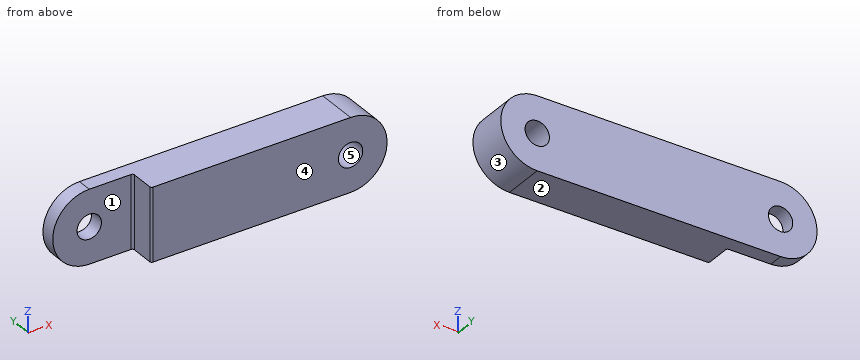
```python
from build123d import *

# Parameters (mm, degrees)
SKETCH1_R           = 2.4
BOSS_EXTRUDE1_DEPTH = 15
SKETCH2_R           = 2.4
CUT_EXTRUDE1_DEPTH  = 12
SKETCH3_W           = 81.763751064
SKETCH3_H           = 26.290001284
CUT_EXTRUDE2_DEPTH  = 5
SCALE1_SCALE        = 0.8
SKETCH4_R           = 2
CUT_EXTRUDE3_DEPTH  = 52.087489074
SKETCH5_W           = 42.014746782
SKETCH5_H           = 19.111045429
CUT_EXTRUDE4_DEPTH  = 1.2
FILLET1_R           = 0.3
FILLET3_R           = 0.3


with BuildPart() as part:
    # Sketch1 → Boss-Extrude1 (new body)
    with BuildSketch(Plane(origin=(0, 0, 0), x_dir=(1, 0, 0), z_dir=(0, 1, 0))):
        with BuildLine():
            Line((-50, 7.5), (0, 7.5))
            ThreePointArc((0, 7.5), (7.5, 0), (0, -7.5))
            Line((0, -7.5), (-50, -7.5))
            ThreePointArc((-50, -7.5), (-57.5, 0), (-50, 7.5))
        make_face()
        with Locations(Location((-50, 0, 0), (0, 0, 270))):
            Circle(SKETCH1_R, mode=Mode.SUBTRACT)
        with Locations(Location((0, 0, 0), (0, 0, 270))):
            Circle(SKETCH1_R, mode=Mode.SUBTRACT)
    extrude(amount=BOSS_EXTRUDE1_DEPTH)

    # Sketch2 → Cut-Extrude1 (cut)
    with BuildSketch(Plane(origin=(0, 0, 0), x_dir=(1, 0, 0), z_dir=(0, 1, 0))):
        with BuildLine():
            Line((-50, 7.5), (-41, 7.5))
            Line((-41, 7.5), (-41, -7.5))
            Line((-41, -7.5), (-50, -7.5))
            ThreePointArc((-50, -7.5), (-57.5, 0), (-50, 7.5))
        make_face()
        with Locations(Location((-50, 0, 0), (0, 0, 270))):
            Circle(SKETCH2_R, mode=Mode.SUBTRACT)
    extrude(amount=CUT_EXTRUDE1_DEPTH, mode=Mode.SUBTRACT)

    # Sketch3 → Cut-Extrude2 (cut)
    with BuildSketch(Plane.XZ):
        with Locations((-24.1072482, 0)):
            Rectangle(SKETCH3_W, SKETCH3_H)
    extrude(amount=-CUT_EXTRUDE2_DEPTH, mode=Mode.SUBTRACT)


with BuildPart() as part_1:
    # Scale1: scaled about (-20.496084793, 10.28858221, 0)
    add(part.part.scale(SCALE1_SCALE).moved(Location((-4.099216959, 2.057716442, 0))))

    # Sketch4 → Cut-Extrude3 (cut, through all)
    with BuildSketch(Plane(origin=(0, 14.057716442, 0), x_dir=(1, 0, 0), z_dir=(0, 1, 0))):
        with Locations(Location((-44.099216959, 0, 0), (0, 0, 270))):
            Circle(SKETCH4_R)
        with Locations(Location((-4.099216959, 0, 0), (0, 0, 270))):
            Circle(SKETCH4_R)
    extrude(amount=-CUT_EXTRUDE3_DEPTH, mode=Mode.SUBTRACT)

    # Sketch5 → Cut-Extrude4 (cut)
    with BuildSketch(Plane.XZ.offset(-6.057716442)):
        with Locations((-17.942307993, -0.717456632)):
            Rectangle(SKETCH5_W, SKETCH5_H)
    extrude(amount=-CUT_EXTRUDE4_DEPTH, mode=Mode.SUBTRACT)

    # Fillet1
    fillet1_edges = [part_1.edges().sort_by_distance(p)[0] for p in [
        (-36.899216959, 11.657716442, 0),
    ]]
    fillet(fillet1_edges, radius=FILLET1_R)

    # Fillet3
    fillet3_edges = [part_1.edges().sort_by_distance(p)[0] for p in [
        (-36.899216959, 7.257716442, 0),
    ]]
    fillet(fillet3_edges, radius=FILLET3_R)


solid = part_1.part
```
Model file for the job. Use its own axes, mm. Face numbers are marked on the shaded views. A direction names the side the tool comes from. Give positions to 0.01 mm unless a question says otherwise; leave off trailing zeros. Order: outer loops, then holes, each group sorted by start corner. A loop starts at its lowest first (then second) coordinate and runs counter-clockwise, first axis right, second up.
1) Saw through at D-D, the plane z = -4.75. Write the cut outline in (x, y), then the cut area to 3 significant figures.
2) 3-axis set-ups, long thin cutter, end or side, ignore diameter. For the marked faces 1 and 2: which of +Z, -Z, +X, -X, +Y, -Y reach the whole face in a straight line?
3) Pin check, flat tips, straight feed: pin 1 (2.5 mm diameter, centred on x = -4.1, z = 0, fed in from +Y); pin 2 (1.5 mm diameter, centred on y = 10.5, z = -1.5, fed in from +X); pin 3 (6.5 mm diameter, centred on x = -44.1, z = 0, fed in from -Y); pin 4 (1.1 mm diameter, centred on y = 9, z = -2.5, fed in from -X). Stop position of each tip, or through.
4) Saw through at B-B, the plane y = 8.5. Write the cut outline in (x, z).
5) Saw through at A-A, the plane z = 0. Write the cut outline in (x, y), then the cut area to 3 significant figures.
6) Mould opens along X. For the marked faces 3, 4 and 5 say: +X half, -X half, draft (parallel to the pull), parting line (faces both ways), or undercut.
7) Wall check: probe 1 along X at (y, z) = (13.3, 0); probe 2 along X at (y, z) = (7.75, 0); probe 3 along Y at (x, z) = (-41, -2). Give the ranges that are in metal, low to high.
8) Saw through at C-C, the plane y = 13.5. Write the cut outline in (x, z), then the cut area to 3 significant figures.
Computed:
1. outline: (-47.76, 11.66) - (-37.2, 11.66) arc R0.3 cw to (-36.9, 11.36) - (-36.9, 7.56) arc R0.3 ccw to (-36.6, 7.26) - (-0.43, 7.26) - (-0.43, 14.06) - (-47.76, 14.06) - close
1. area: 274 mm2
2. face 1: +Z, -Z, -X, -Y
2. face 2: -Z, +X, -X, +Y, -Y
3. pin 1: passes through
3. pin 2: stops at x = 1.85
3. pin 3: stops at y = 11.66
3. pin 4: stops at x = -36.9
4. outline: (-36.9, -6) - (-4.1, -6) arc R6 ccw to (-4.1, 6) - (-36.9, 6) - close; hole circle Ø4 at (-4.1, 0)
5. outline: (-50.1, 11.66) - (-46.1, 11.66) - (-46.1, 14.06) - (-50.1, 14.06) - close; (-42.1, 11.66) - (-37.2, 11.66) arc R0.3 cw to (-36.9, 11.36) - (-36.9, 7.56) arc R0.3 ccw to (-36.6, 7.26) - (-6.1, 7.26) - (-6.1, 14.06) - (-42.1, 14.06) - close; (-2.1, 7.26) - (1.9, 7.26) - (1.9, 14.06) - (-2.1, 14.06) - close
5. area: 259 mm2
6. face 3: +X half
6. face 4: draft
6. face 5: undercut
7. probe 1: x = -50.1 to -46.1, -42.1 to -6.1, -2.1 to 1.9
7. probe 2: x = -36.9 to -6.1, -2.1 to 1.9
7. probe 3: y = 11.66 to 14.06
8. outline: (-44.1, -6) - (-4.1, -6) arc R6 ccw to (-4.1, 6) - (-44.1, 6) arc R6 ccw to start; hole circle Ø4 at (-44.1, 0); hole circle Ø4 at (-4.1, 0)
8. area: 568 mm2
